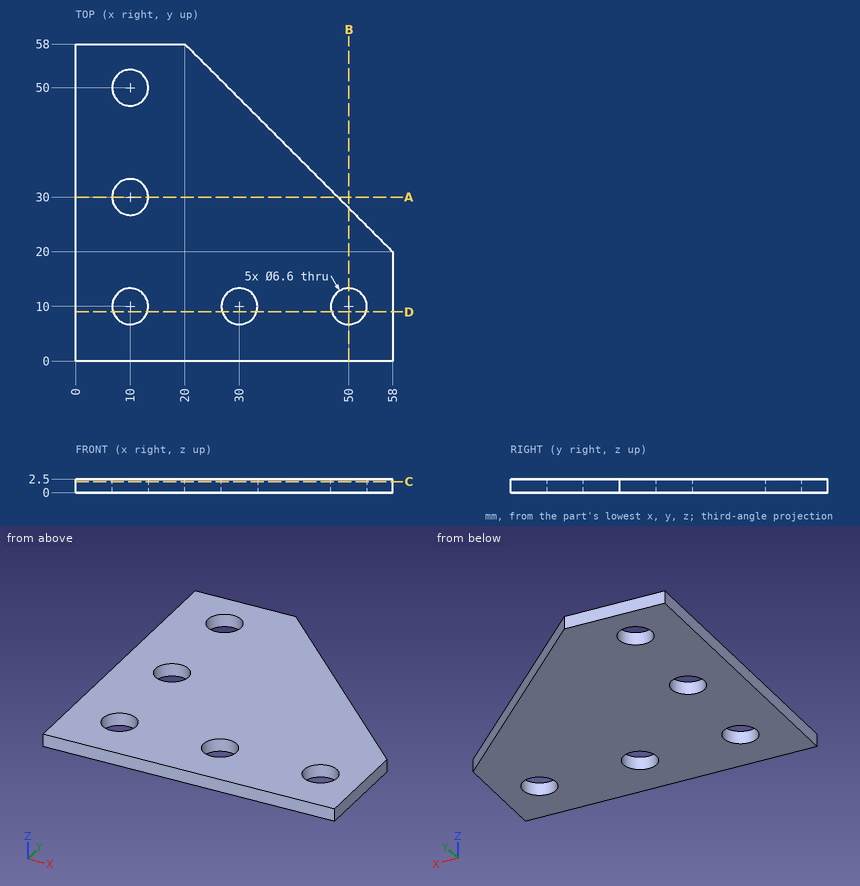
Answer from the drawing. Dimensions are ordinates in mm from the lowest x, y and z of the part. Coordinates: 2 decimals unless noted, no trailing zeros. Loops run counter-clockwise (first coordinate to the right, second up) from the corner with the lowest first, then second, coordinate; pieces in that order, holes last. Notation, with made-up numbers: (68.5, 0.5) - (85.5, 0.5) arc R18 ccw to (85.5, 27.5) - close; hole circle Ø7 at (61, -17). An arc over 180 degrees is marked (long way). Use a Markdown table: item, result.
Item 1: Consider probe 1 along Y at (x, z) = (10, 1.05); probe 2 along X at (y, z) = (11.5, 1.35); probe 3 along Y at (x, z) = (30, 1.75). Determine where each line is inside the solid, lowest interval first. Write a range as from..to.
Evaluation:
| item | result |
|---|---|
| probe 1 | y = 0..6.7, 13.3..26.7, 33.3..46.7, 53.3..58 |
| probe 2 | x = 0..7.06, 12.94..27.06, 32.94..47.06, 52.94..58 |
| probe 3 | y = 0..6.7, 13.3..48 |
Item 2: Find section C-C, the plane z = 2. Determine the outline of the cut face in (x, y), and give its area (3 significant figures).
Evaluation:
| item | result |
|---|---|
| outline | (0, 0) - (58, 0) - (58, 20) - (20, 58) - (0, 58) - close; hole circle Ø6.6 at (10, 10); hole circle Ø6.6 at (10, 30); hole circle Ø6.6 at (10, 50); hole circle Ø6.6 at (30, 10); hole circle Ø6.6 at (50, 10) |
| area | 2,470 mm2 |
Item 3: Given pin 1 Ø6 at (x, y) = (10, 30) entering from -Z, flat-ended and moving along its own axis, determine where the tip first touches the part or whether it passes through.
Evaluation:
| item | result |
|---|---|
| pin 1 | passes through |
Item 4: Find section D-D, the plane y = 9. Determine the outline of the cut face in (x, z), and give its area (3 significant figures).
Evaluation:
| item | result |
|---|---|
| outline | (0, 0) - (6.86, 0) - (6.86, 2.5) - (0, 2.5) - close; (13.14, 0) - (26.86, 0) - (26.86, 2.5) - (13.14, 2.5) - close; (33.14, 0) - (46.86, 0) - (46.86, 2.5) - (33.14, 2.5) - close; (53.14, 0) - (58, 0) - (58, 2.5) - (53.14, 2.5) - close |
| area | 97.8 mm2 |
Item 5: Find section B-B, the plane x = 50. Determine the outline of the cut face in (y, z), and give its area (3 significant figures).
Evaluation:
| item | result |
|---|---|
| outline | (0, 0) - (6.7, 0) - (6.7, 2.5) - (0, 2.5) - close; (13.3, 0) - (28, 0) - (28, 2.5) - (13.3, 2.5) - close |
| area | 53.5 mm2 |
Item 6: Find section A-A, the plane y = 30. Determine the outline of the cut face in (x, z).
Evaluation:
| item | result |
|---|---|
| outline | (0, 0) - (6.7, 0) - (6.7, 2.5) - (0, 2.5) - close; (13.3, 0) - (48, 0) - (48, 2.5) - (13.3, 2.5) - close |
